```python
from build123d import *

# Parameters (mm, degrees)
SKETCH1_R           = 10
BOSS_EXTRUDE1_DEPTH = 95
SKETCH3_R           = 14.99
BOSS_EXTRUDE2_DEPTH = 85
CHAMFER1_SIZE       = 1


with BuildPart() as part:
    # Sketch1 → Boss-Extrude1 (new body, symmetric)
    with BuildSketch(Plane(origin=(0, 0, 0), x_dir=(1, 0, 0), z_dir=(0, 1, 0))):
        Circle(SKETCH1_R)
    extrude(amount=BOSS_EXTRUDE1_DEPTH, both=True)

    # Sketch3 → Boss-Extrude2 (add)
    with BuildSketch(Plane(origin=(0, -70, 0), x_dir=(-1, 0, 0), z_dir=(0, -1, 0))):
        Circle(SKETCH3_R)
    extrude(amount=-BOSS_EXTRUDE2_DEPTH)

    # Chamfer1
    chamfer1_edges = [part.edges().sort_by_distance(p)[0] for p in [
        (-10, 95, 0),
    ]]
    chamfer(chamfer1_edges, length=CHAMFER1_SIZE)


solid = part.part
```
Model file for the job. Use its own axes, mm. A direction names the side the tool comes from. Coordinates: 2 decimals unless noted, no trailing zeros. Write each loop counter-clockwise with the first axis right and the second up, starting at its lowest first coordinate (ties: lowest second). Pieces come first, ordered by that corner, then holes. Notation, with made-up numbers: (0.5, 11.5) - (58.5, 11.5) arc R13 ccw to (58.5, 21.5) - close; hole circle Ø6 at (-25, 5). An arc over 180 degrees is marked (long way). Use a Markdown table: item, result. Add a question column.
Item 1: Drop flat-ended pins along their axis: pin 1 (6 mm diameter, centred on x = 7.5, y = -58, fed in from -Z); pin 2 (10 mm diameter, centred on y = 52, z = -6, fed in from +X); pin 3 (10 mm diameter, centred on y = 57, z = 2, fed in from -X); pin 4 (4 mm diameter, centred on y = -33, z = 1.5, fed in from -X). Give the stop position or say it passes through.
Item 2: Band-saw the part on B-B, the plane z = 0. Write the cut outline in (x, y), and give its area (3 significant figures).
Item 3: Band-saw the part on D-D, the plane y = 70. Write the cut outline in (x, z).
Item 4: Drill centre lines: line 1 along Y through (x, z) = (-4.25, 11.5); line 2 along Z through (x, y) = (0, 25.5); line 3 along Z through (x, y) = (-1.25, 3.5). Where is each one in solid material? Low to high.
Item 5: 3-axis set-ups, long thin cutter, end or side, ignore diameter. For faces 1 (the face through (0, -95, 0)), 2 (the face through (-2.17, -82.32, 9.76)), 3 (the face through (-2.17, 55.05, 9.76)): which of +Z, -Z, +X, -X, +Y, -Y reach the whole face in a straight line?
Item 6: Band-saw the part on A-A, the plane x = 0. Write the cut outline in (y, z).
Item 7: Band-saw the part on C-C, the plane y = -19. Write the cut outline in (x, z).
A:
| question | item | result |
|---|---|---|
| 1 | pin 1 | stops at z = -14.3 |
| 1 | pin 2 | stops at x = 9.95 |
| 1 | pin 3 | stops at x = -10 |
| 1 | pin 4 | stops at x = -14.99 |
| 2 | outline | (-14.99, -70) - (-10, -70) - (-10, -95) - (10, -95) - (10, -70) - (14.99, -70) - (14.99, 15) - (10, 15) - (10, 94) - (9, 95) - (-9, 95) - (-10, 94) - (-10, 15) - (-14.99, 15) - close |
| 2 | area | 4,650 mm² |
| 3 | outline | circle Ø20 at (0, 0) |
| 4 | line 1 | y = -70 to 15 |
| 4 | line 2 | z = -10 to 10 |
| 4 | line 3 | z = -14.94 to 14.94 |
| 5 | face 1 | +Z, -Z, +X, -X, -Y |
| 5 | face 2 | -Y |
| 5 | face 3 | +Y |
| 6 | outline | (-95, -10) - (-70, -10) - (-70, -14.99) - (15, -14.99) - (15, -10) - (94, -10) - (95, -9) - (95, 9) - (94, 10) - (15, 10) - (15, 14.99) - (-70, 14.99) - (-70, 10) - (-95, 10) - close |
| 7 | outline | circle Ø29.98 at (0, 0) |
